Source: CAD feature listing. Evaluate the final solid. Frame: model axes, mm. Round coordinates to 2 decimals unless told otherwise and drop trailing zeros. Order: outer loops, then holes, each group sorted by start corner. A loop starts at its lowest first (then second) coordinate and runs counter-clockwise, first axis right, second up. Notation, with made-up numbers: (50, 85.25) - (60, 85.25) arc R18 cw to (60, 99.25) - close; hole circle Ø4 at (52, 40.5). An arc over 180 degrees is marked (long way). Return JSON: item names as keys, results as strings. Group by question number.
1) Contact query for flat-ended pins moving along their axis: P1, Ø10, axis at y = -27, z = -8.5, coming from the -X side; P2, Ø6, axis at x = 6.5, y = -16, coming from the +Z side; P3, Ø1.6, axis at x = 1, y = -93.5, coming from the -Z side. Output: stop coordinate, or through.
2) Section D-D, the plane x = 2.5. Return loops of the section in (y, z), plus the area to 3 significant figures.
3) Section C-C, the plane y = -45.5. Return loops of the section in (x, z), plus the area to 3 significant figures.
4) Section B-B, the plane z = 5.25. Return loops of the section in (x, y).
5) Section A-A, the plane x = -5.5. Return loops of the section in (y, z).
6) Ray query, line 1 (Y direction, x = -2.5, z = -4.5); line 2 (X direction, y = -62, z = 0.5). Return the intervals inside material, ascending. Write a range as from..to.
```python
from build123d import *

# Parameters (mm, degrees)
F0_R     = 11
F1_DEPTH = 95
F2_W     = 12.7
F2_H     = 4.7625
F2_W_2   = 7.5
F2_H_2   = 2.5
F3_DEPTH = 2


# Not quite as in the source:
# - a feature names something its author has since deleted; it is built from what else it names


with BuildPart() as f1:
    # F0 (on Front) → F1 (new body)
    with BuildSketch(Plane.XZ):
        Circle(F0_R)
    extrude(amount=F1_DEPTH)

    # F2 (on face) → F3 (cut)
    with BuildSketch(Plane.XZ.offset(95)):
        with Locations((0, 4.6411268625)):
            Rectangle(F2_W, F2_H)
        with Locations((0, -4.4527297777)):
            Rectangle(F2_W_2, F2_H_2)
    extrude(amount=-F3_DEPTH, mode=Mode.SUBTRACT)


solid = f1.part
```
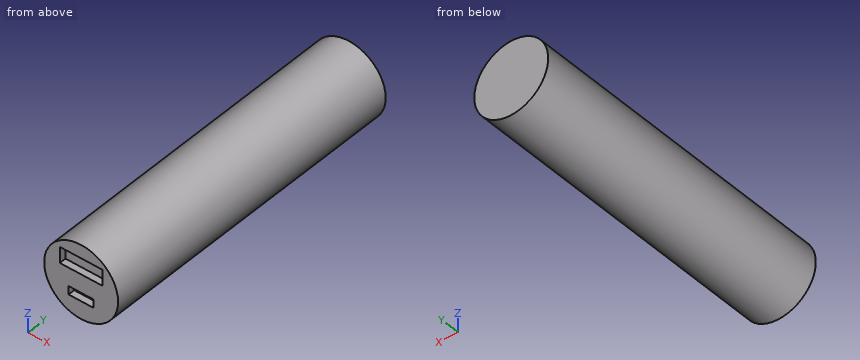
Geometry check:
{
 "1": {"P1": "x = -10.43", "P2": "z = 10.43", "P3": "z = -11"},
 "2": {"outline": "(-95, -10.71) - (0, -10.71) - (0, 10.71) - (-95, 10.71) - (-95, 7.02) - (-93, 7.02) - (-93, 2.26) - (-95, 2.26) - (-95, -3.2) - (-93, -3.2) - (-93, -5.7) - (-95, -5.7) - close", "area": "2,020 mm2"},
 "3": {"outline": "circle Ø22 at (0, 0)", "area": "380 mm2"},
 "4": {"outline": "(-9.67, -95) - (-6.35, -95) - (-6.35, -93) - (6.35, -93) - (6.35, -95) - (9.67, -95) - (9.67, 0) - (-9.67, 0) - close"},
 "5": {"outline": "(-95, -9.53) - (0, -9.53) - (0, 9.53) - (-95, 9.53) - (-95, 7.02) - (-93, 7.02) - (-93, 2.26) - (-95, 2.26) - close"},
 "6": {"line 1": "-93..0", "line 2": "-10.99..10.99"}
}
